Part model, mm, in its own coordinate system. A direction names the side the tool comes from. Round coordinates to 2 decimals unless told otherwise and drop trailing zeros. Order: outer loops, then holes, each group sorted by start corner. A loop starts at its lowest first (then second) coordinate and runs counter-clockwise, first axis right, second up. Notation, with made-up numbers: M 24,-36 L 60,-36 A13 ccw 60,-21 Z; hole C 15,79 d5. An arc over 180 degrees is marked long. Write each question's results on one line, items separated by ' | '. Start each with the question number.
1. Band-saw the part on B-B, the plane z = -6.5. List the corners of the cut face in (x, y).
2. Probe L1, parallel to Y at x = 0, z = -7.2; L2, parallel to X at y = 0, z = -4.75. List the from-to ranges inside material, lowest first. Write a range as [from, to].
3. Band-saw the part on A-A, the plane z = 0.75. List the corners of the cut face in (x, y).
4. Drop flat-ended pins along their axis: pin 1 Ø3 at (x, y) = (2.5, -12.5) entering from -Z; pin 2 Ø4 at (x, z) = (-3.5, -1) entering from +Y; pin 3 Ø4 at (y, z) = (3, -5) entering from -X. Give the stop position or say it passes through.
5. Two-plate mould, pull along X, no slides. Class faces 6 (the face through (17, 14, -0.615)), 7 (the face through (-5.794, -0.255, -6.45)), 8 (the face through (-2.994, -22.804, 2.493)): +X half, -X half, draft (parallel to the pull), parting line (faces both ways), or undercut.
6. Which spindle directions (+Z, -Z, +X, -X, +Y, -Y) get a long thin tool onto all of the face, cutting with end or side? Do faces 1 (the face through (-2.17, 9.76, -5.41)), 2 (the face through (-2.994, -22.804, -8.307)), 3 (the face through (-4.3, 4.3, -8.915)), 4 (the face through (-2.799, -21.317, 0.652)), 5 (the face through (2.4, -0.1, 0)). Say none if no direction does.
```python
from build123d import *

# Parameters (mm, degrees)
F2_R     = 2.25
F3_DEPTH = 8.916156


with BuildPart() as f1:
    # F0 (on Front) → F1 (revolve)
    with BuildSketch(Plane.XZ):
        with BuildLine():
            Line((4.850819, 0), (0, 0))
            Line((0, 0), (0, -1.915156))
            ThreePointArc((0, -1.915156), (3.067572, -2.429197), (5.8, -3.915156))
            Line((5.8, -3.915156), (5.8, -8.915156))
            Line((5.8, -8.915156), (10, -8.915156))
            Line((10, -8.915156), (10, -2))
            Line((10, -2), (18.356489, -2))
            Line((18.356489, -2), (18.356489, -8.915156))
            Line((18.356489, -8.915156), (23, -8.915156))
            Line((23, -8.915156), (23, -7.715156))
            Line((23, -7.715156), (21.5, -7.715156))
            Line((21.5, -7.715156), (21.5, -5.215156))
            Line((21.5, -5.215156), (23, -5.215156))
            Line((23, -5.215156), (23, -0.615156))
            Line((23, -0.615156), (21.5, -0.615156))
            Line((21.5, -0.615156), (21.5, 1.884844))
            Line((21.5, 1.884844), (23, 1.884844))
            Line((23, 1.884844), (23, 3.084844))
            Line((23, 3.084844), (20.772453, 3.084844))
            Line((20.772453, 3.084844), (19.854128, -0.925569))
            Line((19.854128, -0.925569), (19.694118, 0))
            ThreePointArc((19.694118, 0), (14.847059, 4.035723), (10, 0))
            ThreePointArc((10, 0), (7.801044, 1.972172), (5.602089, 0))
            Line((5.602089, 0), (4.850819, 0))
        make_face()
    revolve(axis=Axis((0, 0, -0.957578), (0, 0, -1)))

    # F2 (on face) → F3 (cut, through all)
    with BuildSketch(Plane.XY):
        Circle(F2_R)
    extrude(amount=-F3_DEPTH, mode=Mode.SUBTRACT)


solid = f1.part
```
Solution:
1) outline: C 0,0 d43; C 0,0 d20; hole C 0,0 d36.71; hole C 0,0 d11.6
2) L1: [-21.5, -18.36], [-10, -5.8], [5.8, 10], [18.36, 21.5] | L2: [-23, -18.36], [-10, -5.8], [5.8, 10], [18.36, 23]
3) outline: C 0,0 d43; C 0,0 d38.99; C 0,0 d19.56; hole C 0,0 d40.48; hole C 0,0 d20.4; hole C 0,0 d11.65
4) pin 1: z = -2 | pin 2: y = 22.95 | pin 3: x = -22.98
5) face 6: draft | face 7: undercut | face 8: parting line
6) face 1: -Z | face 2: +Z, -Z | face 3: -Z, +X, -X, +Y, -Y | face 4: none | face 5: +Z
